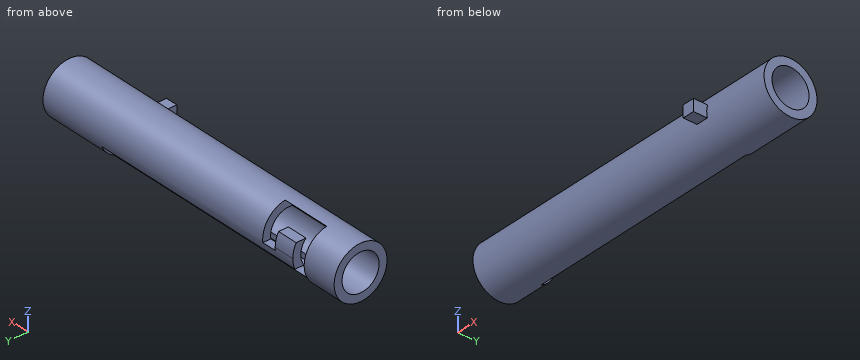
Autodesk Inventor part; units mm, degrees
ref_plane "YZ Plane" through (0, 0, 0) normal (1, 0, 0) x (0, 1, 0)
ref_plane "XY Plane" through (0, 0, 0) normal (0, 0, 1) x (1, 0, 0)
sketch "Schizzo2" plane through (0, 0, 0) normal (1, 0, 0) x (0, 1, 0)
  circle A0 centre (0, -11) radius 10
  point P0 (0, 0)
  dimension "d4" = 11
  dimension "d5" = 20
extrude "Estrusione1" add sketch "Schizzo2" against normal blind 128
shell "Svuotamento1" thickness 3 removed faces 2 at (0, -3.2365, -10.2023) at (-128, -3.2365, -10.2023)
sketch "Schizzo1" plane through (0, 0, 0) normal (0, 1, 0) x (-1, 0, 0)
  line L0 (0, 0) -> (0, -20)
  line L1 (0, -10) -> (128, -10)
  line L2 (128, 0) -> (128, -20)
  line L3 (0, -20) -> (25, -20)
  line L4 (25, -20) -> (128, -20)
  line L5 (128, 0) -> (0, 0)
  dimension "d0" = 20
  dimension "d3" = 25
ref_plane "Piano di lavoro7" through (0, 10, -11) normal (0, 1, 0) x (-1, 0, 0)
sketch "Schizzo13" plane through (0, 10, -11) normal (0, 1, 0) x (-1, 0, 0)
  line L0 (24.8317, -9) -> (114.8317, -9)
  line L1 (24.8317, -9) -> (24.8317, -4)
  line L2 (24.8317, -4) -> (109.8317, -4)
  line L3 (114.8317, -9) -> (114.8317, 9.8878)
  line L4 (0, 7) -> (128, 7)
  line L5 (109.8317, -4) -> (109.8317, 4.8878)
  line L6 (114.8317, 9.8878) -> (96.5899, 9.8878)
  line L7 (96.5899, 9.8878) -> (96.5899, -1.1122)
  line L8 (96.5899, -1.1122) -> (102.0899, -1.1122)
  line L9 (102.0899, -1.1122) -> (102.0899, 4.8878)
  line L10 (109.8317, 4.8878) -> (102.0899, 4.8878)
  point P0 (0, 11)
  dimension "d59" = 90
  dimension "d60" = 5
  dimension "d61" = 85
  dimension "d62" = 6
  dimension "d63" = 5
  dimension "d64" = 5.5
  dimension "d65" = 11
extrude "Estrusione7" cut sketch "Schizzo13" against normal blind 11.25
ref_plane "Piano di lavoro8" through (0, -10, -11) normal (0, 1, 0) x (-1, 0, 0)
sketch "Schizzo14" plane through (0, -10, -11) normal (0, 1, 0) x (-1, 0, 0)
  line L0 (25.2013, -2.0707) -> (29.7013, -2.0707)
  line L1 (29.7013, -2.0707) -> (29.7013, 2.4293)
  line L2 (29.7013, 2.4293) -> (25.2013, 2.4293)
  line L3 (25.2013, 2.4293) -> (25.2013, -2.0707)
  point P0 (0, 11)
  dimension "d68" = 4.5
  dimension "d69" = 4.5
extrude "Estrusione8" add sketch "Schizzo14" along normal blind 2.5 and the other way blind 5
properties part number "astaoscilla2_306"
Input: part model. Units: mm. Frame: model coordinates. Coordinates: 2 decimals unless noted, no trailing zeros. Loops run counter-clockwise (first coordinate to the right, second up) from the corner with the lowest first, then second, coordinate; pieces in that order, holes last. Notation, with made-up numbers: (32, 8.25) -> (49, 8.25) arc R4 cw to (49, 14.25) -> close; hole circle Ø3 at (-31, 53.25). An arc over 180 degrees is marked (long way). Write item = value, one per line. Start each with the question number.
Item 1: Cut plane B-B, the plane x = -21. Return loops of the section in (y, z), plus the area to 3 significant figures.
Item 2: Cut plane A-A, the plane y = 0. Return loops of the section in (x, z).
Item 3: Cut plane C-C, the plane x = -86.5. Return loops of the section in (y, z), plus the area to 3 significant figures.
Item 4: Material intervals for line 1 (X direction, y = 6.25, z = -17.75); line 2 (Z direction, x = -34.5, y = 0); line 3 (Y direction, x = -93, z = -11.5), sorted ascending.
Item 5: First-contact query: P1, Ø2.5, axis at x = -80.5, z = -18.5, coming from the +Y side; P2, Ø3.5, axis at x = -28, y = -13, coming from the +Z side; P3, Ø2.5, axis at x = -98, y = 9, coming from the +Z side. Flat tips, straight axial feed; report the tip coordinate or a pass-through.
Ans:
q1.outline = circle Ø20 at (0, -11); hole circle Ø14 at (0, -11)
q1.area = 160 mm²
q2.outline = (-128, -21) -> (0, -21) -> (0, -18) -> (-24.83, -18) -> (-24.83, -20) -> (-114.83, -20) -> (-114.83, -18) -> (-128, -18) -> close; (-128, -4) -> (-114.83, -4) -> (-114.83, -1.11) -> (-96.59, -1.11) -> (-96.59, -4) -> (0, -4) -> (0, -1) -> (-128, -1) -> close
q3.outline = (-1.25, -20) -> (-1.25, -17.89) arc R7 cw (long way) to (5.74, -15) -> (9.17, -15) arc R10 ccw (long way) to (4.36, -20) -> close
q3.area = 133 mm²
q4.line_1 = -128 to -114.83, -24.83 to 0
q4.line_2 = -21 to -20, -4 to -1
q4.line_3 = -9.99 to -6.98, 6.98 to 9.99
q5.P1 = -1.25
q5.P2 = -8.57
q5.P3 = -12.11
